Here's how the part is built. I have some questions about the finished solid (model axes, mm). A direction names the side the tool comes from. Round coordinates to 2 decimals unless told otherwise and drop trailing zeros. Write each loop counter-clockwise with the first axis right and the second up, starting at its lowest first coordinate (ties: lowest second). Pieces come first, ordered by that corner, then holes. Notation, with made-up numbers: (68, -31) - (125, -31) arc R13 cw to (125, -21) - close; hole circle Ø2 at (22, -38.75). An arc over 180 degrees is marked (long way). Use one line per item in the form item = value. Start each with the question number.
1. Will these pins go through, and if not, where does the flat tip stop? pin 1 (2 mm diameter, centred on x = -128, z = 178.5, fed in from -Y); pin 2 (7.5 mm diameter, centred on x = -46.5, y = -155, fed in from +Z); pin 3 (5 mm diameter, centred on y = -157.5, z = 112.5, fed in from -X).
2. Which directions (+Z, -Z, +X, -X, +Y, -Y) give clear straight access to the entire face, cutting with the end or side of a thin tool? Please do faces 1 (the flat face through (15.02, -157, 114)), 2 (the flat face through (-33, -157, 124.872)), 3 (the flat face through (-79.138, -157, 114)).
3. I want a section at B-B, the plane x = -122. List the corners of the cut face in (y, z) for me.
4. If I drill on line 1 along Y through (x, z) = (-18, 31.5); line 2 along Y through (x, z) = (12.5, 106); line 3 along Z through (x, y) = (-137, -150), over which ranges is the centre line in solid material (lowest first)?
5. I want a section at D-D, the plane x = -59. List the corners of the cut face in (y, z) for me (3 decimals).
6. I want a section at C-C, the plane z = 153. List the corners of the cut face in (x, y) for me.
```python
from build123d import *

# Parameters (mm, degrees)
F0_W     = 203.2
F0_H     = 254
F1_DEPTH = 152.4
F2_R     = 5.08
F3_W     = 94.158622
F3_H     = 21.369308
F4_DEPTH = 12.7
F5_R     = 3.175


with BuildPart() as f1:
    # F0 (on Front) → F1 (new body)
    with BuildSketch(Plane.XZ):
        with Locations((-70.276403, 113.863483)):
            Rectangle(F0_W, F0_H)
    extrude(amount=F1_DEPTH)

    # F2
    f2_edges = [f1.edges().sort_by_distance(p)[0] for p in [
        (-70.276403, -152.4, 240.863483),
        (31.323597, -76.2, 240.863483),
        (-171.876403, -76.2, 240.863483),
        (-70.276403, 0, 240.863483),
        (31.323597, -152.4, 113.863483),
        (-171.876403, -152.4, 113.863483),
        (-70.276403, -152.4, -13.136517),
        (31.323597, -76.2, -13.136517),
        (-171.876403, -76.2, -13.136517),
    ]]
    fillet(f2_edges, radius=F2_R)

    # F3 (on face) → F4 (join)
    with BuildSketch(Plane.XZ.offset(152.4)):
        with Locations((-32.059189, 114.187598)):
            Rectangle(F3_W, F3_H)
    extrude(amount=F4_DEPTH)

    # F5
    f5_edges = [f1.edges().sort_by_distance(p)[0] for p in [
        (-32.059189, -165.1, 103.502944),
        (15.020122, -165.1, 114.187598),
        (-32.059189, -165.1, 124.872252),
        (-79.1385, -165.1, 114.187598),
    ]]
    fillet(f5_edges, radius=F5_R)


solid = f1.part
```
Model answer:
q1.pin_1 = -152.4
q1.pin_2 = 239
q1.pin_3 = -79.14
q2.face_1 = +Z, -Z, +X, -Y
q2.face_2 = +Z, +X, -X, -Y
q2.face_3 = +Z, -Z, -X, -Y
q3.outline = (-152.4, -8.06) arc R5.08 ccw to (-147.32, -13.14) - (0, -13.14) - (0, 235.78) arc R5.08 ccw to (-5.08, 240.86) - (-147.32, 240.86) arc R5.08 ccw to (-152.4, 235.78) - close
q4.line_1 = -152.4 to 0
q4.line_2 = -165.03 to 0
q4.line_3 = -12.37 to 240.1
q5.outline = (-165.1, 106.678) arc R3.175 ccw to (-161.925, 103.503) - (-152.4, 103.503) - (-152.4, -8.057) arc R5.08 ccw to (-147.32, -13.137) - (0, -13.137) - (0, 235.783) arc R5.08 ccw to (-5.08, 240.863) - (-147.32, 240.863) arc R5.08 ccw to (-152.4, 235.783) - (-152.4, 124.872) - (-161.925, 124.872) arc R3.175 ccw to (-165.1, 121.697) - close
q6.outline = (-171.88, -147.32) arc R5.08 ccw to (-166.8, -152.4) - (26.24, -152.4) arc R5.08 ccw to (31.32, -147.32) - (31.32, 0) - (-171.88, 0) - close
